Design review of the part built by this model. Coordinates are the model's own, in mm. Face numbers are marked on the shaded views. A direction names the side the tool comes from. Give positions to 0.01 mm unless a question says otherwise; leave off trailing zeros. Loops run counter-clockwise (first coordinate to the right, second up) from the corner with the lowest first, then second, coordinate; pieces in that order, holes last.
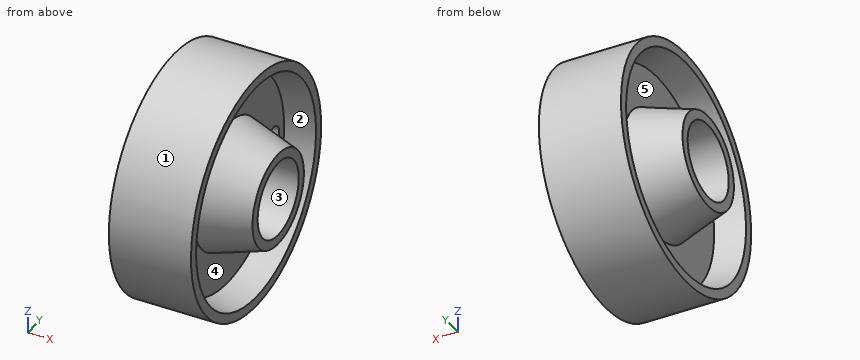
from build123d import *

# Parameters (mm, degrees)
CUT_EXTRUDE1_DEPTH      = 67.992536898
CUT_EXTRUDE1_DEPTH_BACK = 67.992536898
SKETCH2_R               = 12
CUT_EXTRUDE2_DEPTH      = 59.855755878
CUT_EXTRUDE2_DEPTH_BACK = 59.855755878
SKETCH3_R               = 3.185465226


with BuildPart() as part:
    # Sketch1 → Revolve1 (revolve)
    with BuildSketch(Plane.XY, mode=Mode.PRIVATE) as revolve1_sk:
        Polygon((-13, 38), (13, 38), (13, 35), (4, 33), (4, 20), (20, 15), (20, 0), (-20, 0), (-20, 15), (-4, 20), (-4, 33), (-13, 35), align=None)
    revolve(revolve1_sk.sketch.rotate(Axis((-115.826136374, 0, 0), (1, 0, 0)), 90), axis=Axis((-115.826136374, 0, 0), (1, 0, 0)))

    # Sketch2 → Cut-Extrude1 (cut, two sides: drawn at the far end of the back side and taken through both)
    with BuildSketch(Plane(origin=(20, 0, 0), x_dir=(0, 0, -1), z_dir=(1, 0, 0)).offset(-CUT_EXTRUDE1_DEPTH_BACK)):
        Circle(SKETCH2_R)
    extrude(amount=CUT_EXTRUDE1_DEPTH + CUT_EXTRUDE1_DEPTH_BACK, mode=Mode.SUBTRACT)

    # Sketch3 → Cut-Extrude2 (cut, two sides: drawn at the far end of the back side and taken through both)
    with BuildSketch(Plane(origin=(4, 0, 0), x_dir=(0, 0, -1), z_dir=(1, 0, 0)).offset(-CUT_EXTRUDE2_DEPTH_BACK)):
        with Locations((0, 26.917181157)):
            Circle(SKETCH3_R)
    extrude(amount=CUT_EXTRUDE2_DEPTH + CUT_EXTRUDE2_DEPTH_BACK, mode=Mode.SUBTRACT)


solid = part.part
Q1. Draft analysis for pull direction Z (two halves, no side actions). For the marked faces 1 and 2, state which applies: pulls with the +Z half, pulls with the -Z half, needs draft (parallel to the pull), parting line crosses it, or undercut.
Results:
face 1: parting line crosses it
face 2: undercut
Q2. Take a section at B-B (z = 0). Give the boundary of the cut face in (x, y).
Results:
outline: (-20, -15) - (-4, -20) - (-4, -33) - (-13, -35) - (-13, -38) - (13, -38) - (13, -35) - (4, -33) - (4, -20) - (20, -15) - (20, -12) - (-20, -12) - close; (-20, 12) - (20, 12) - (20, 15) - (4, 20) - (4, 23.73) - (-4, 23.73) - (-4, 20) - (-20, 15) - close; (-13, 35) - (-4, 33) - (-4, 30.1) - (4, 30.1) - (4, 33) - (13, 35) - (13, 38) - (-13, 38) - close
Q3. Tool access review of the marked faces 3, 4 and 5: name each direction out of +Z, -Z, +X, -X, +Y, -Y from which nothing blocks a thin tool from reaching the whole face with its end or side.
Results:
face 3: +X, -X
face 4: +X
face 5: -X
Q4. Insertion check: pin 1 (3 mm diameter, centred on y = -21.5, z = 2.5, fed in from +X); pin 2 (10 mm diameter, centred on x = -3, z = 15, fed in from +Y); pin 3 (4 mm diameter, centred on y = 26.92, z = 0, fed in from -X); pin 4 (5 mm diameter, centred on x = 9.5, y = -17, fed in from -Z). Each pin has a flat end and moves straight along its axis. Give the tip position at first contact, or say it passes through.
Results:
pin 1: stops at x = 4
pin 2: stops at y = 36.66
pin 3: passes through
pin 4: stops at z = -35.12
Q5. Wall thickness on line 1 (Y direction, x = 0, z = 0); line 2 (Z direction, x = -9, y = -5); line 3 (Y direction, x = 12, z = -11): over which ranges is each line inside the solid? List them lowest first.
Results:
line 1: y = -38 to -12, 12 to 23.73, 30.1 to 38
line 2: z = -37.67 to -33.74, -17.75 to -10.91, 10.91 to 17.75, 33.74 to 37.67
line 3: y = -36.37 to -32.99, -13.61 to -4.8, 4.8 to 13.61, 32.99 to 36.37
Q6. Take a section at A-A (y = 0). Give the boundary of the cut face in (x, z).
Results:
outline: (-20, -15) - (-4, -20) - (-4, -33) - (-13, -35) - (-13, -38) - (13, -38) - (13, -35) - (4, -33) - (4, -20) - (20, -15) - (20, -12) - (-20, -12) - close; (-20, 12) - (20, 12) - (20, 15) - (4, 20) - (4, 33) - (13, 35) - (13, 38) - (-13, 38) - (-13, 35) - (-4, 33) - (-4, 20) - (-20, 15) - close
Q7. Take a section at C-C (x = -3). Give the boundary of the cut face in (y, z).
Results:
outline: circle Ø76 at (0, 0); hole circle Ø24 at (0, 0); hole circle Ø6.37 at (26.92, 0)
